The figure shows three views and two pictorial views of one solid part (mm, origin at its lowest corner). Answer the questions. Coordinates: 2 decimals unless noted, no trailing zeros. Order: outer loops, then holes, each group sorted by start corner. A loop starts at its lowest first (then second) coordinate and runs counter-clockwise, first axis right, second up. Notation, with made-up numbers: (-10, 26.5) - (20, 26.5) arc R18 ccw to (20, 39.5) - close; hole circle Ø1 at (-38.5, -21.75). An arc over 180 degrees is marked (long way). Answer as a JSON object with one key per item and string values. Group by question number.
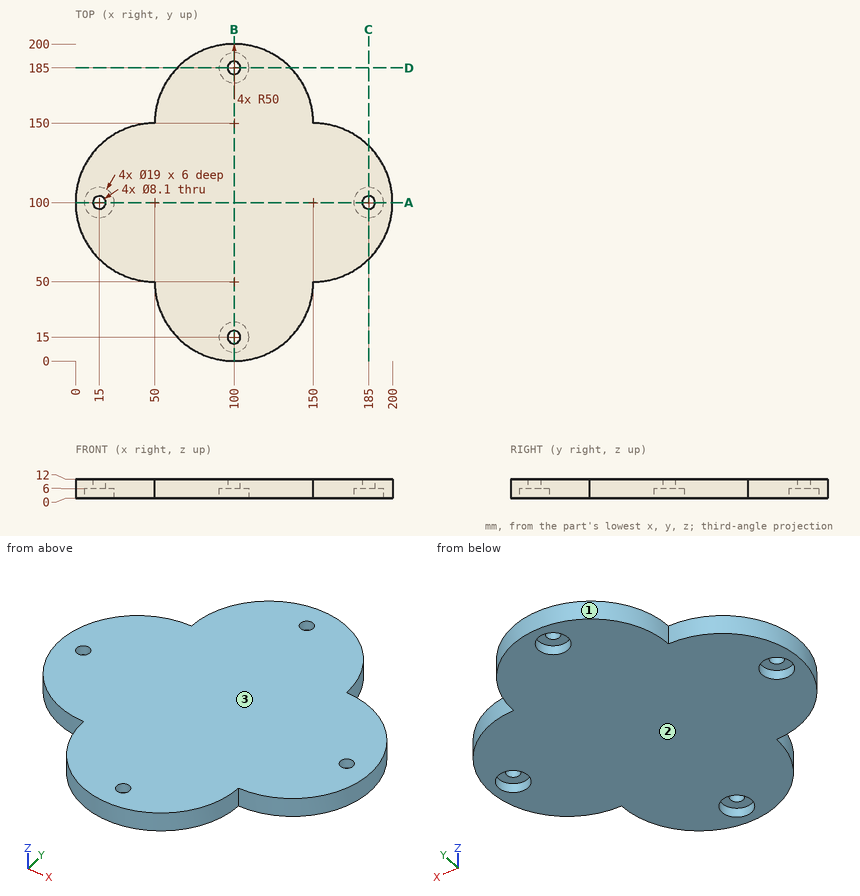
1. A cutting plane is placed at C-C on x = 185. Write down the section's boundary in (y, z).
2. For a pull along Z with two mould halves and no side action, classify the marked faces 1, 2 and 3 as pulls with the +Z half, pulls with the -Z half, needs draft (parallel to the pull), parting line crosses it, or undercut.
3. A cutting plane is placed at A-A on y = 100. Write down the section's boundary in (x, z).
4. Given pin 1 (5 mm diameter, centred on x = 140.5, z = 9.5, fed in from -Y); pin 2 (7.5 mm diameter, centred on x = 100, y = 15, fed in from -Z); pin 3 (5.5 mm diameter, centred on x = 104.5, y = 187.5, fed in from -Z); pin 4 (4 mm diameter, centred on x = 65.5, z = 9.5, fed in from +Y), each flat-ended and moving along its own axis, determine where each tip first touches the part or whether it passes through.
5. Straight lines are drawn through the part: L1, parallel to X at y = 103, z = 7; L2, parallel to X at y = 188, z = 7; L3, parallel to X at y = 185, z = 7.95. For each, find the intervals that lie inside material, in ascending order.
Derived:
{
 "1": {"outline": "(64.29, 0) - (90.5, 0) - (90.5, 6) - (95.95, 6) - (95.95, 12) - (64.29, 12) - close; (104.05, 6) - (109.5, 6) - (109.5, 0) - (135.71, 0) - (135.71, 12) - (104.05, 12) - close"},
 "2": {"face 1": "needs draft", "face 2": "pulls with the -Z half", "face 3": "pulls with the +Z half"},
 "3": {"outline": "(0, 0) - (5.5, 0) - (5.5, 6) - (10.95, 6) - (10.95, 12) - (0, 12) - close; (19.05, 6) - (24.5, 6) - (24.5, 0) - (175.5, 0) - (175.5, 6) - (180.95, 6) - (180.95, 12) - (19.05, 12) - close; (189.05, 6) - (194.5, 6) - (194.5, 0) - (200, 0) - (200, 12) - (189.05, 12) - close"},
 "4": {"pin 1": "stops at y = 17.5", "pin 2": "passes through", "pin 3": "stops at z = 6", "pin 4": "stops at y = 188"},
 "5": {"L1": "x = 0.09 to 12.28, 17.72 to 182.28, 187.72 to 199.91", "L2": "x = 67.5 to 97.28, 102.72 to 132.5", "L3": "x = 64.29 to 95.95, 104.05 to 135.71"}
}
